from build123d import *

# Parameters (mm, degrees)
SKETCH_1_W      = 26.7
SKETCH_1_H      = 24.3
SKETCH_1_R      = 1.5
EXTRUDE_1_DEPTH = 3
SKETCH_2_R      = 1
EXTRUDE_2_DEPTH = 3
EXTRUDE_3_DEPTH = 8


with BuildPart() as part:
    # 草图1 → 凸台-拉伸1 (new body)
    with BuildSketch(Plane.XY):
        with Locations((20.044402297, 0)):
            Rectangle(SKETCH_1_W, SKETCH_1_H)
        with Locations((30.499402297, 9.375)):
            Circle(SKETCH_1_R, mode=Mode.SUBTRACT)
        with Locations((9.589402297, 9.375)):
            Circle(SKETCH_1_R, mode=Mode.SUBTRACT)
        with Locations((30.499402297, -9.375)):
            Circle(SKETCH_1_R, mode=Mode.SUBTRACT)
        with Locations((9.589402297, -9.375)):
            Circle(SKETCH_1_R, mode=Mode.SUBTRACT)
    extrude(amount=EXTRUDE_1_DEPTH)

    # 草图2 → 凸台-拉伸2 (add)
    with BuildSketch(Plane.XY.offset(3)):
        with BuildLine():
            Line((12.044402297, 8), (18.544402297, 8))
            Line((18.544402297, 8), (18.544402297, 10.65))
            ThreePointArc((18.544402297, 10.65), (20.044402297, 12.15), (21.544402297, 10.65))
            Line((21.544402297, 10.65), (21.544402297, 8))
            Line((21.544402297, 8), (28.044402297, 8))
            Line((28.044402297, 8), (28.044402297, 1.75))
            Line((28.044402297, 1.75), (28.044402297, -1.75))
            Line((28.044402297, -1.75), (28.044402297, -8))
            Line((28.044402297, -8), (21.544402297, -8))
            Line((21.544402297, -8), (21.544402297, -10.65))
            ThreePointArc((21.544402297, -10.65), (20.044402297, -12.15), (18.544402297, -10.65))
            Line((18.544402297, -10.65), (18.544402297, -8))
            Line((18.544402297, -8), (12.044402297, -8))
            Line((12.044402297, -8), (12.044402297, -1.75))
            Line((12.044402297, -1.75), (12.044402297, 1.75))
            Line((12.044402297, 1.75), (12.044402297, 8))
        make_face()
        with Locations((20.044402297, 10.65)):
            Circle(SKETCH_2_R, mode=Mode.SUBTRACT)
        with Locations((20.044402297, -10.65)):
            Circle(SKETCH_2_R, mode=Mode.SUBTRACT)
    extrude(amount=EXTRUDE_2_DEPTH)

    # 草图3 → 凸台-拉伸3 (add)
    with BuildSketch(Plane.XY.offset(6)):
        with BuildLine():
            Line((27.935532249, 1.315320523), (28.709062769, 1.315320523))
            Line((28.709062769, 1.315320523), (28.709062769, -1.315320523))
            Line((28.709062769, -1.315320523), (27.935532249, -1.315320523))
            ThreePointArc((27.935532249, -1.315320523), (12.044402297, 0), (27.935532249, 1.315320523))
        make_face()
    extrude(amount=EXTRUDE_3_DEPTH)


solid = part.part
Geometry check sheet. Reference: the model listing, model coordinates, mm. A direction names the side the tool comes from. Round coordinates to 2 decimals unless told otherwise and drop trailing zeros. Write each loop counter-clockwise with the first axis right and the second up, starting at its lowest first coordinate (ties: lowest second). Pieces come first, ordered by that corner, then holes.
Item 1: Section check C-C (y = -10). Record the boundary of the cut face in (x, z).
Determined:
outline: (6.69, 0) - (8.23, 0) - (8.23, 3) - (6.69, 3) - close; (10.95, 0) - (29.14, 0) - (29.14, 3) - (21.54, 3) - (21.54, 6) - (20.8, 6) - (20.8, 3) - (19.28, 3) - (19.28, 6) - (18.54, 6) - (18.54, 3) - (10.95, 3) - close; (31.86, 0) - (33.39, 0) - (33.39, 3) - (31.86, 3) - close
Item 2: Section check A-A (x = 29.5). Record the boundary of the cut face in (y, z).
Determined:
outline: (-12.15, 0) - (-10.49, 0) - (-10.49, 3) - (-12.15, 3) - close; (-8.26, 0) - (8.26, 0) - (8.26, 3) - (-8.26, 3) - close; (10.49, 0) - (12.15, 0) - (12.15, 3) - (10.49, 3) - close
Item 3: Mould release check, pull along Y, two halves, no side actions. Record for faces 1 (the face through (20.1, 8.4, 6)), 2 (the face through (25, 8, 4)), 3 (the face through (20, 11, 3)), 4 (the face through (19.91, 11.64, 4.48)): +Y half, -Y half, draft (parallel to the pull), parting line (faces both ways), or undercut.
Determined:
face 1: draft
face 2: +Y half
face 3: undercut
face 4: undercut
Item 4: Section check D-D (z = 2.5). Record the boundary of the cut face in (x, y) (3 decimals), plus the area to 3 significant figures.
Determined:
outline: (6.694, -12.15) - (33.394, -12.15) - (33.394, 12.15) - (6.694, 12.15) - close; hole circle Ø3 at (9.589, -9.375); hole circle Ø3 at (9.589, 9.375); hole circle Ø3 at (30.499, -9.375); hole circle Ø3 at (30.499, 9.375)
area: 621 mm2
Item 5: Section check B-B (z = 4.5). Record the boundary of the cut face in (x, y), plus the area to 3 significant figures.
Determined:
outline: (12.04, -8) - (18.54, -8) - (18.54, -10.65) arc R1.5 ccw to (21.54, -10.65) - (21.54, -8) - (28.04, -8) - (28.04, 8) - (21.54, 8) - (21.54, 10.65) arc R1.5 ccw to (18.54, 10.65) - (18.54, 8) - (12.04, 8) - close; hole circle Ø2 at (20.04, -10.65); hole circle Ø2 at (20.04, 10.65)
area: 273 mm2
Item 6: Access from +Z, -Z, +X, -X, +Y, -Y to the whole of each face (thin tool, end or side, straight path). Record for faces 5 (the face through (12.05, -0.33, 9.94)), 6 (the face through (18.544, -9, 4)), 7 (the face through (12.044, 0, 4)), 8 (the face through (20.01, 12.15, 4.48)), 9 (the face through (28.709, 0, 10)).
Determined:
face 5: +Z
face 6: +Z, -X, -Y
face 7: +Z, -X, +Y, -Y
face 8: +Z, +Y
face 9: +Z, +X, +Y, -Y
Item 7: Material ranges on line 1 along Z through (x, y) = (28, -7); line 2 along X through (y, z) = (3.5, 4.5); line 3 along Z through (x, y) = (9.5, -7.25), recorded low to high.
Determined:
line 1: z = 0 to 6
line 2: x = 12.04 to 28.04
line 3: z = 0 to 3
Item 8: Go/stop test with flat-tipped pins: pin 1 Ø0.9 at (x, z) = (24.5, 4) entering from -Y; pin 2 Ø1.3 at (y, z) = (0, 11.5) entering from +X; pin 3 Ø2.5 at (x, z) = (23.5, 4.5) entering from +Y. Record where each tip stops, or that it passes through.
Determined:
pin 1: stops at y = -8
pin 2: stops at x = 28.71
pin 3: stops at y = 8
